CAD build for the part. Positions are in the model's coordinates, mm. A direction names the side the tool comes from. Give positions to 0.01 mm unless a question says otherwise; leave off trailing zeros. Order: outer loops, then holes, each group sorted by start corner. A loop starts at its lowest first (then second) coordinate and runs counter-clockwise, first axis right, second up.
from build123d import *

# Parameters (mm, degrees)
SKETCH1_W             = 13
SKETCH1_H             = 1
BOSS_EXTRUDE1_DEPTH   = 6
BOSS_EXTRUDE1_2_DEPTH = 6
SKETCH1_3_W           = 13
SKETCH1_3_H           = 12.1
BOSS_EXTRUDE2_DEPTH   = 1
SKETCH2_W             = 2
SKETCH2_H             = 14.1
BOSS_EXTRUDE3_DEPTH   = 4
CHAMFER1_SIZE         = 1
CUT_EXTRUDE1_DEPTH    = 2.5


with BuildPart() as part:
    # Sketch1 → Boss-Extrude1 (new body)
    with BuildSketch(Plane.XY):
        with Locations((0, 6.55)):
            Rectangle(SKETCH1_W, SKETCH1_H)
    extrude(amount=BOSS_EXTRUDE1_DEPTH)



with BuildPart() as body_2:
    # Sketch1 → Boss-Extrude1 2 (new body)
    with BuildSketch(Plane.XY):
        with Locations((0, -6.55)):
            Rectangle(SKETCH1_W, SKETCH1_H)
    extrude(amount=BOSS_EXTRUDE1_2_DEPTH)


with BuildPart() as part_1:
    add(part.part)

    add(body_2.part)  # Boss-Extrude2 merges body 2
    # Sketch1<3> → Boss-Extrude2 (add)
    with BuildSketch(Plane.XY):
        Rectangle(SKETCH1_3_W, SKETCH1_3_H)
    extrude(amount=BOSS_EXTRUDE2_DEPTH)

    # Sketch2 → Boss-Extrude3 (add)
    with BuildSketch(Plane(origin=(0, 0, 0), x_dir=(-1, 0, 0), z_dir=(0, 0, -1))):
        with Locations((5.5, 0)):
            Rectangle(SKETCH2_W, SKETCH2_H)
        Polygon((-6.5, -3.05), (-2.6, -3.55), (-2.6, -7.05), (-6.5, -7.05), align=None)
        Polygon((-6.5, 7.05), (-2.6, 7.05), (-2.6, 3.55), (-6.5, 3.05), align=None)
    extrude(amount=BOSS_EXTRUDE3_DEPTH)

    # Chamfer1
    chamfer1_edges = [part_1.edges().sort_by_distance(p)[0] for p in [
        (-6.5, -7.05, 1),
        (6.5, -7.05, 1),
        (-6.5, 7.05, 1),
        (6.5, 7.05, 1),
    ]]
    chamfer(chamfer1_edges, length=CHAMFER1_SIZE - 0.0001)  # a hair under: the kernel refuses the full size

    # Sketch3 → Cut-Extrude1 (cut)
    with BuildSketch(Plane.ZY.offset(-2.6)):
        Polygon((-1, -7.05), (-4, -4.55), (-4, -7.05), align=None)
        Polygon((-1, 7.05), (-4, 4.55), (-4, 7.05), align=None)
    extrude(amount=-CUT_EXTRUDE1_DEPTH, mode=Mode.SUBTRACT)


solid = part_1.part
1. 3-axis set-ups, long thin cutter, end or side, ignore diameter. For faces 4 (the flat face through (3.8, 5.8, -2.5)), 5 (the flat face through (5.4, -4.6, -4)), 6 (the flat face through (4.523, 3.303, -1.972)), 7 (the flat face through (0, 6.05, 3)), 8 (the flat face through (-4.5, 0, -2)): which of +Z, -Z, +X, -X, +Y, -Y reach the whole face in a straight line?
2. Wall check: line 1 (Y direction, x = -0.75, z = 3); line 2 (X direction, y = 3.75, z = -0.75); line 3 (Z direction, x = -1.25, y = 2). Give the ranges that are in metal, low to high.
3. Mould opens along X. For faces 1 (the flat face through (0, 7.05, 3)), 2 (the flat face through (3.8, -5.8, -2.5)), 3 (the flat face through (-6.5, 0, -2)) say: released by +X, released by -X, zero draft, split by the parting line, or undercut.
4. Saw through at C-C on z = -1.25. Give the cut face in (x, y).
5. Saw through at D-D on x = -1.5. Give the cut face in (y, z).
6. Pin check, flat tips, straight feed: P1, Ø2, axis at y = -2, z = -1.5, coming from the +X side; P2, Ø2, axis at x = 4.5, y = 0.5, coming from the -Z side; P3, Ø1.5, axis at x = 4.5, y = 2, coming from the +Z side. Stop position of each tip, or through.
7. Saw through at B-B on y = -5.25. Give the cut face in (x, z), plus the area to 3 significant figures.
Reported:
1. face 4: -Z, +Y
1. face 5: -Z, +X, -X, +Y, -Y
1. face 6: -Z
1. face 7: +Z, +X, -X
1. face 8: -Z, +Y, -Y
2. line 1: y = -7.05 to -6.05, 6.05 to 7.05
2. line 2: x = -6.5 to -4.5, 2.6 to 6.5
2. line 3: z = 0 to 1
3. face 1: zero draft
3. face 2: undercut
3. face 3: released by -X
4. outline: (-6.5, -6.05) - (-5.5, -7.05) - (-4.5, -7.05) - (-4.5, 7.05) - (-5.5, 7.05) - (-6.5, 6.05) - close; (2.6, -6.84) - (5.1, -6.84) - (5.1, -7.05) - (5.5, -7.05) - (6.5, -6.05) - (6.5, -3.05) - (2.6, -3.55) - close; (2.6, 3.55) - (6.5, 3.05) - (6.5, 6.05) - (5.5, 7.05) - (5.1, 7.05) - (5.1, 6.84) - (2.6, 6.84) - close
5. outline: (-7.05, 0) - (7.05, 0) - (7.05, 6) - (6.05, 6) - (6.05, 1) - (-6.05, 1) - (-6.05, 6) - (-7.05, 6) - close
6. P1: stops at x = -4.5
6. P2: stops at z = 0
6. P3: stops at z = 1
7. outline: (-6.5, -4) - (-4.5, -4) - (-4.5, 0) - (2.6, 0) - (2.6, -3.16) - (5.1, -3.16) - (5.1, -4) - (6.5, -4) - (6.5, 1) - (-6.5, 1) - close
7. area: 34.5 mm2
